from build123d import *

# Parameters (mm, degrees)
SKETCH1_W           = 34
SKETCH1_H           = 20
BOSS_EXTRUDE1_DEPTH = 20.5
SKETCH2_OUTSIDE_W   = 47.378
SKETCH2_OUTSIDE_H   = 33.378
SKETCH2_OUTSIDE_W_2 = 32.9
SKETCH2_OUTSIDE_H_2 = 19
CUT_EXTRUDE2_DEPTH  = 45.204072211
CUT_EXTRUDE5_DEPTH  = 20.5
SKETCH3_W           = 0.125
SKETCH3_H           = 13
CUT_EXTRUDE3_DEPTH  = 25
CHAMFER1_SIZE       = 0.85
CHAMFER2_SIZE       = 0.85
CHAMFER3_SIZE       = 1
CHAMFER4_SIZE       = 1
BOSS_EXTRUDE2_DEPTH = 2
SKETCH10_R          = 3
BOSS_EXTRUDE3_DEPTH = 6
FILLET1_R           = 2
SCALE_1_SCALE       = 1.7


with BuildPart() as part:
    # Sketch1 → Boss-Extrude1 (new, symmetric)
    with BuildSketch(Plane(origin=(0, 0, 0), x_dir=(0, 0, -1), z_dir=(1, 0, 0))):
        with Locations((0, 14)):
            Rectangle(SKETCH1_W, SKETCH1_H)
    extrude(amount=BOSS_EXTRUDE1_DEPTH, both=True)

    # Sketch2 outside → Cut-Extrude2 (cut, through all)
    with BuildSketch(Plane(origin=(12.5, 0, 0), x_dir=(0, 0, -1), z_dir=(1, 0, 0))):
        with Locations((0, 14)):
            Rectangle(SKETCH2_OUTSIDE_W, SKETCH2_OUTSIDE_H)
        with Locations((0, 13.5)):
            Rectangle(SKETCH2_OUTSIDE_W_2, SKETCH2_OUTSIDE_H_2, mode=Mode.SUBTRACT)
    cut_extrude2 = extrude(amount=CUT_EXTRUDE2_DEPTH, mode=Mode.SUBTRACT)

    # Mirror1: Cut-Extrude2 across plane
    add(cut_extrude2.mirror(Plane(origin=(0, 0, 0), x_dir=(0, 0, 1), z_dir=(1, 0, 0))), mode=Mode.SUBTRACT)

    # Sketch5 → Cut-Extrude5 (cut, symmetric)
    with BuildSketch(Plane(origin=(0, 0, 0), x_dir=(0, 0, -1), z_dir=(1, 0, 0))):
        with BuildLine():
            Line((-6.5, 12.5), (-7.5, 11.5))
            Line((-7.5, 11.5), (-7.5, 10))
            ThreePointArc((-7.5, 10), (-7.220600207, 9.128142709), (-6.486486487, 8.581081081))
            ThreePointArc((-6.486486487, 8.581081081), (-5.059724667, 5.990862007), (-7.5, 4.320550528))
            Line((-7.5, 4.320550528), (-7.5, 0.5))
            Line((-7.5, 0.5), (-7, 0))
            Line((-7, 0), (7, 0))
            Line((7, 0), (7.5, 0.5))
            Line((7.5, 0.5), (7.5, 4.320550528))
            ThreePointArc((7.5, 4.320550528), (5.059724667, 5.990862007), (6.486486487, 8.581081081))
            ThreePointArc((6.486486487, 8.581081081), (7.220600207, 9.128142709), (7.5, 10))
            Line((7.5, 10), (7.5, 11.5))
            Line((7.5, 11.5), (6.5, 12.5))
            Line((6.5, 12.5), (-6.5, 12.5))
        make_face()
    extrude(amount=CUT_EXTRUDE5_DEPTH, both=True, mode=Mode.SUBTRACT)

    # Sketch3 → Cut-Extrude3 (cut)
    with BuildSketch(Plane(origin=(12.5, 0, 0), x_dir=(0, 0, -1), z_dir=(1, 0, 0))):
        with Locations((-16.9375, 10.5)):
            Rectangle(SKETCH3_W, SKETCH3_H)
    cut_extrude3 = extrude(amount=-CUT_EXTRUDE3_DEPTH, mode=Mode.SUBTRACT)

    # Mirror2: Cut-Extrude3 across plane
    add(cut_extrude3.mirror(Plane.XY), mode=Mode.SUBTRACT)

    # Chamfer1
    chamfer1_edges = [part.edges().sort_by_distance(p)[0] for p in [
        (16.5, 23, -16.45),
        (16.5, 23, 16.45),
        (-16.5, 23, 16.45),
        (-16.5, 23, -16.45),
    ]]
    chamfer(chamfer1_edges, length=CHAMFER1_SIZE)

    # Chamfer2
    chamfer2_edges = [part.edges().sort_by_distance(p)[0] for p in [
        (0, 24, 17),
        (0, 24, -17),
    ]]
    chamfer(chamfer2_edges, length=CHAMFER2_SIZE)

    # Chamfer3
    chamfer3_edges = [part.edges().sort_by_distance(p)[0] for p in [
        (16.5, 4, 16.45),
        (16.5, 4, -16.45),
        (-16.5, 4, -16.45),
        (-16.5, 4, 16.45),
    ]]
    chamfer(chamfer3_edges, length=CHAMFER3_SIZE)

    # Chamfer4
    chamfer4_edges = [part.edges().sort_by_distance(p)[0] for p in [
        (0, 4, 16.875),
        (0, 4, -16.875),
    ]]
    chamfer(chamfer4_edges, length=CHAMFER4_SIZE)

    # Sketch7 → Boss-Extrude2 (add)
    with BuildSketch(Plane(origin=(20.5, 0, 0), x_dir=(0, 0, -1), z_dir=(1, 0, 0))):
        Polygon((-2.020725942, 15.5), (2.020725942, 15.5), (4.041451884, 19), (2.020725942, 22.5), (-2.020725942, 22.5), (-4.041451884, 19), align=None)
    extrude(amount=BOSS_EXTRUDE2_DEPTH)

    # Sketch9 → Cut-Revolve1 (revolve, cut)
    with BuildSketch(Plane.XY):
        Polygon((22.5, 22.75), (21.5, 23.803780125), (20.5, 22.75), (20.5, 24), (22.5, 24), align=None)
    revolve(axis=Axis((20.5, 19, 0), (1, 0, 0)), mode=Mode.SUBTRACT)

    # Sketch10 → Boss-Extrude3 (add)
    with BuildSketch(Plane(origin=(20.5, 0, 0), x_dir=(0, 0, -1), z_dir=(1, 0, 0))):
        with Locations((0, 19)):
            Circle(SKETCH10_R)
    extrude(amount=BOSS_EXTRUDE3_DEPTH)

    # Fillet1
    fillet1_edges = [part.edges().sort_by_distance(p)[0] for p in [
        (26.5, 19, 3),
    ]]
    fillet(fillet1_edges, radius=FILLET1_R)


with BuildPart() as part_1:
    # Scale 1: scaled about (0, 0, 0)
    add(part.part.scale(SCALE_1_SCALE))


solid = part_1.part
Build history of the part. All positions in model axes, mm. A direction names the side the tool comes from. Round coordinates to 2 decimals unless told otherwise and drop trailing zeros. Loops run counter-clockwise (first coordinate to the right, second up) from the corner with the lowest first, then second, coordinate; pieces in that order, holes last. Notation, with made-up numbers: (-13, -19.5) -> (14, -19.5) arc R17 ccw to (14, -15.5) -> close; hole circle Ø1 at (35.5, 14.5). An arc over 180 degrees is marked (long way). Use CSV: the item, a comma, the result in double quotes. Start each with the question number.
Q1. Saw through at A-A on x = 30. Give the cut face in (y, z) (3 decimals), and give its area (3 significant figures).
Q2. Which spindle directions (+Z, -Z, +X, -X, +Y, -Y) get a long thin tool onto all of the face, cutting with end or side? Do faces 5 (the face through (27.955, 7.662, 27.127)), 6 (the face through (-28, 23, -27.965)), 7 (the face through (-28, 23, 27.965)), 8 (the face through (0, 19, 28.688)), 9 (the face through (0.5, 20.4, -11.9)). Say none if no direction does.
Q3. Mould opens along Y. For faces 1 (the face through (28, 39.1, 0)), 2 (the face through (-27.955, 7.662, -27.127)), 3 (the face through (0, 34, 28.9)), 4 (the face through (0.49, 15.54, 12.29)) say: +Y half, -Y half, draft (parallel to the pull), parting line (faces both ways), or undercut.
Q4. Saw through at B-B on z = 21.5. Give the cut face in (x, y).
Q5. Drill centre lines: L1, parallel to Z at x = 9.5, y = 17.5; L2, parallel to Y at x = 31.5, z = 20; L3, parallel to X at y = 30, z = -15.5. Where is each one in solid material? Low to high.
Q6. Flat gauge pins, fed straight in: pin 1 Ø4 at (x, y) = (-26.5, 27.5) entering from +Z (3 decimals); pin 2 Ø4 at (x, y) = (-30.5, 16.5) entering from -Z (3 decimals); pin 3 Ø10 at (x, y) = (5, 18.5) entering from -Z. Where does each tip first touch, or does it go through?
Solutions:
1,outline,"(6.8, -26.265) -> (8.5, -27.965) -> (37.655, -27.965) -> (39.1, -26.52) -> (39.1, 26.52) -> (37.655, 27.965) -> (8.5, 27.965) -> (6.8, 26.265) -> (6.8, 12.75) -> (7.345, 12.75) arc R3.74 ccw to (14.588, 11.027) arc R2.55 cw to (17, 12.75) -> (19.55, 12.75) -> (21.25, 11.05) -> (21.25, -11.05) -> (19.55, -12.75) -> (17, -12.75) arc R2.55 cw to (14.588, -11.027) arc R3.74 ccw to (7.345, -12.75) -> (6.8, -12.75) -> close"
1,area,"1,490 mm^2"
2,face 5,"+Z, +X, -Y"
2,face 6,"-Z, -X, +Y, -Y"
2,face 7,"+Z, -X, +Y, -Y"
2,face 8,"+Z, +X, -X, -Y"
2,face 9,"+X, -X"
3,face 1,"+Y half"
3,face 2,"-Y half"
3,face 3,"draft"
3,face 4,"undercut"
4,outline,"(-34.85, 6.8) -> (34.85, 6.8) -> (34.85, 39.1) -> (21.25, 39.1) -> (21.25, 40.8) -> (-21.25, 40.8) -> (-21.25, 39.1) -> (-34.85, 39.1) -> close"
5,L1,"z = -28.69 to -12.75, 12.75 to 28.69"
5,L2,"y = 6.8 to 39.1"
5,L3,"x = -34.85 to 34.85"
6,pin 1,"stops at z = 27.965"
6,pin 2,"stops at z = -27.965"
6,pin 3,"stops at z = -28.69"
